```python
from build123d import *

# Parameters (mm, degrees)
SKETCH2_R           = 3.175
BOSS_EXTRUDE1_DEPTH = 3.175
FILLET1_R           = 5.08


with BuildPart() as part:
    # Sketch2 → Boss-Extrude1 (new, symmetric)
    with BuildSketch(Plane(origin=(0, 0, 0), x_dir=(1, 0, 0), z_dir=(0, 1, 0))):
        with BuildLine():
            Line((-19.05, 6.35), (-19.05, -25.4))
            Line((-19.05, -25.4), (19.05, -25.4))
            Line((19.05, -25.4), (19.05, 6.35))
            ThreePointArc((19.05, 6.35), (13.470384188, 19.820384175), (1.9e-08, 25.4))
            ThreePointArc((1.9e-08, 25.4), (-13.470384175, 19.820384188), (-19.05, 6.35))
        make_face()
        with Locations(Location((0, -19.05, 0), (0, 0, 270))):
            Circle(SKETCH2_R, mode=Mode.SUBTRACT)
        with BuildLine():
            ThreePointArc((-5.715, 0.635), (-11.43, 6.35), (-5.715, 12.065))
            Line((-5.715, 12.065), (5.715, 12.065))
            ThreePointArc((5.715, 12.065), (11.43, 6.35), (5.715, 0.635))
            Line((5.715, 0.635), (-5.715, 0.635))
        make_face(mode=Mode.SUBTRACT)
    extrude(amount=BOSS_EXTRUDE1_DEPTH, both=True)

    # Fillet1
    fillet1_edges = [part.edges().sort_by_distance(p)[0] for p in [
        (19.05, -1.5875, 25.4),
        (-19.05, -1.5875, 25.4),
    ]]
    fillet(fillet1_edges, radius=FILLET1_R)


solid = part.part
```
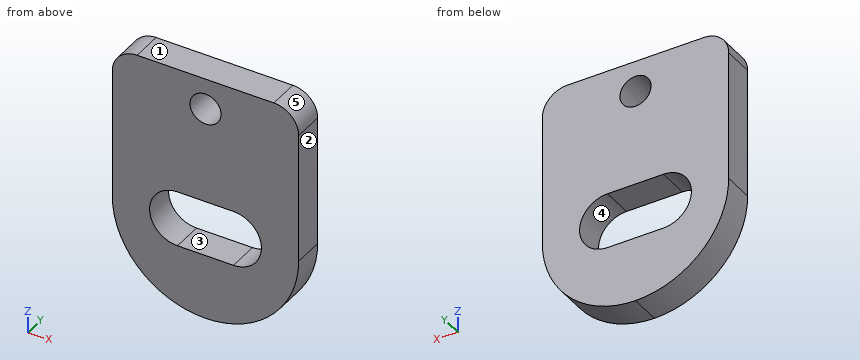
Check sheet for the modelled part. Datum: model origin and axes. Units: mm. Face numbers are marked on the shaded views. A direction names the side the tool comes from. Give positions to 0.01 mm unless a question says otherwise; leave off trailing zeros. Loops run counter-clockwise (first coordinate to the right, second up) from the corner with the lowest first, then second, coordinate; pieces in that order, holes last. Notation, with made-up numbers: M 68,16.25 L 99,16.25 A12 cw 99,38.25 Z; hole C 31.5,-20 d4. An arc over 180 degrees is marked long. Answer in a Markdown table with one row per item.
1) Depth check by flat-ended pin: pin 1 (2 mm diameter, centred on x = 5, y = -0.5, fed in from -Z). Enter the tip coordinate at first touch or a pass-through.
Solutions:
| item | result |
|---|---|
| pin 1 | stops at z = -24.98 |
2) Tool access check on the marked faces 4 and 5. Record the directions out of +Z, -Z, +X, -X, +Y, -Y that give a thin tool (end or side, any length) a straight path to the whole face; none if there is none.
Solutions:
| item | result |
|---|---|
| face 4 | +Y, -Y |
| face 5 | +Z, +X, +Y, -Y |
3) Cross-section at A-A (y = -0.75). Enter the section's corners in (x, z) (3 decimals), plus the area to 3 significant figures.
Solutions:
| item | result |
|---|---|
| outline | M -19.05,-6.35 A19.05 ccw 19.05,-6.35 L 19.05,20.32 A5.08 ccw 13.97,25.4 L -13.97,25.4 A5.08 ccw -19.05,20.32 Z; hole M -5.715,-12.065 L 5.715,-12.065 A5.715 ccw 5.715,-0.635 L -5.715,-0.635 A5.715 ccw Z; hole C 0,19.05 d6.35 |
| area | 1,500 mm^2 |
4) Thickness scan on line 1 (Z direction, x = -2.5, y = 0.5) (3 decimals); line 2 (Z direction, x = 1, y = 1.25) (3 decimals); line 3 (X direction, y = -0.25, z = 19.05) (3 decimals). Record the ranges inside material, lowest first.
Solutions:
| item | result |
|---|---|
| line 1 | z = -25.235 to -12.065, -0.635 to 17.093, 21.007 to 25.4 |
| line 2 | z = -25.374 to -12.065, -0.635 to 16.037, 22.063 to 25.4 |
| line 3 | x = -19.05 to -3.175, 3.175 to 19.05 |
5) Cross-section at C-C (x = -8). Enter the section's corners in (y, z) (3 decimals).
Solutions:
| item | result |
|---|---|
| outline | M -3.175,-23.639 L 3.175,-23.639 L 3.175,-11.588 L -3.175,-11.588 Z; M -3.175,-1.112 L 3.175,-1.112 L 3.175,25.4 L -3.175,25.4 Z |
6) Cross-section at D-D (x = -13). Enter the section's corners in (y, z) (3 decimals), plus the area to 3 significant figures.
Solutions:
| item | result |
|---|---|
| outline | M -3.175,-20.275 L 3.175,-20.275 L 3.175,25.4 L -3.175,25.4 Z |
| area | 290 mm^2 |
7) Cross-section at B-B (z = 19.05). Enter the section's corners in (x, y) (3 decimals).
Solutions:
| item | result |
|---|---|
| outline | M -19.05,-3.175 L -3.175,-3.175 L -3.175,3.175 L -19.05,3.175 Z; M 3.175,-3.175 L 19.05,-3.175 L 19.05,3.175 L 3.175,3.175 Z |
8) Mould release check, pull along Z, two halves, no side actions. Record for the marked faces 1, 2 and 3: released by +Z, released by -Z, zero draft, split by the parting line, or undercut.
Solutions:
| item | result |
|---|---|
| face 1 | released by +Z |
| face 2 | zero draft |
| face 3 | undercut |
